Geometry: see drawing. Coordinates: mm, zero at the bounding-box minimum. A direction names the side the tool comes from. Round coordinates to 2 decimals unless told otherwise and drop trailing zeros. Write each loop counter-clockwise with the first axis right and the second up, starting at its lowest first coordinate (ties: lowest second). Pieces come first, ordered by that corner, then holes. Notation, with made-up numbers: M -12.75,0 L 11.25,0 A21 cw 11.25,37 Z; hole C -36,46 d11. An arc over 180 degrees is marked long. Use one line per item in the form item = value. Start each with the question number.
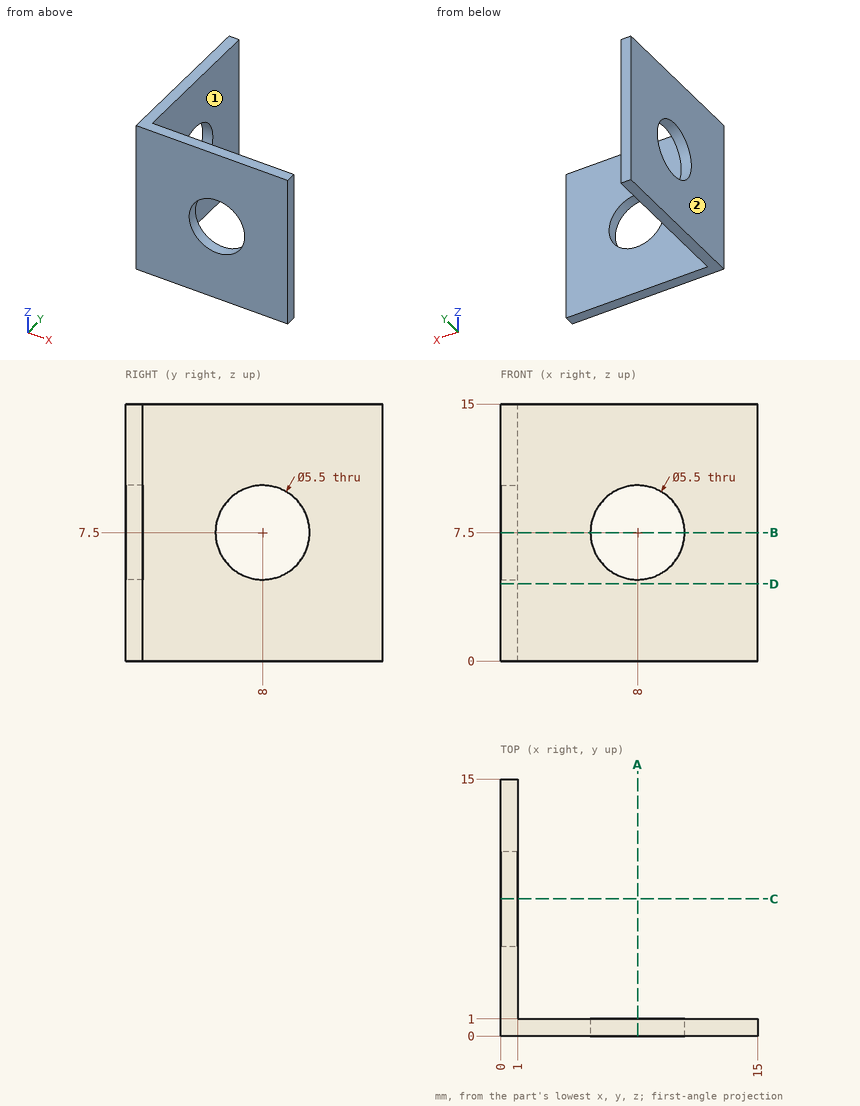
Item 1: First-contact query: pin 1 (6 mm diameter, centred on y = 5, z = 7, fed in from +X); pin 2 (8 mm diameter, centred on x = 5, y = 3, fed in from +Z); pin 3 (7 mm diameter, centred on x = 9, z = 9.5, fed in from +Y). Flat tips, straight axial feed; report the tip coordinate or a pass-through.
Item 2: Cut plane A-A (x = 8). Output: boundary loops of the cut face in (y, z).
Item 3: Ray query, line 1 (Z direction, x = 8, y = 0.4); line 2 (Y direction, x = 11.25, z = 9.5). Return the intervals inside material, ascending. Write a range as from..to.
Item 4: Reachability of the marked faces 1 and 2 from +Z, -Z, +X, -X, +Y, -Y: full face, straight path, thin tool, end or side. Return the list, or none.
Item 5: Cut plane B-B (z = 7.5). Output: boundary loops of the cut face in (x, y), plus the area to 3 significant figures.
Item 6: Cut plane D-D (z = 4.5). Output: boundary loops of the cut face in (x, y).
Final values:
q1.pin_1 = 1
q1.pin_2 = 15
q1.pin_3 = 1
q2.outline = M 0,0 L 1,0 L 1,4.75 L 0,4.75 Z; M 0,10.25 L 1,10.25 L 1,15 L 0,15 Z
q3.line_1 = 0..4.75, 10.25..15
q3.line_2 = 0..1
q4.face_1 = +Z, -Z, +X, +Y
q4.face_2 = +Z, -Z, -X, +Y, -Y
q5.outline = M 0,0 L 5.25,0 L 5.25,1 L 1,1 L 1,5.25 L 0,5.25 Z; M 0,10.75 L 1,10.75 L 1,15 L 0,15 Z; M 10.75,0 L 15,0 L 15,1 L 10.75,1 Z
q5.area = 18.0 mm^2
q6.outline = M 0,0 L 15,0 L 15,1 L 1,1 L 1,15 L 0,15 Z
